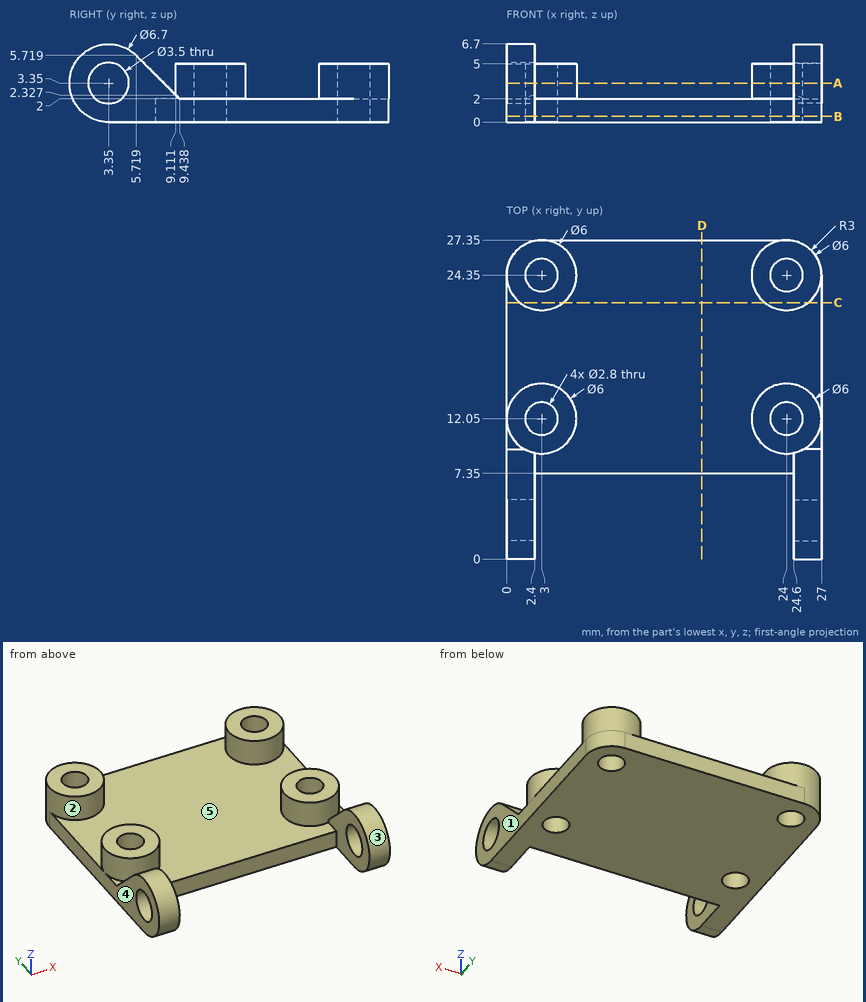
Source: three-view drawing plus pictorial views. Frame: mm from the lowest corner of the part. A direction names the side the tool comes from. Round coordinates to 2 decimals unless told otherwise and drop trailing zeros. Order: outer loops, then holes, each group sorted by start corner. A loop starts at its lowest first (then second) coordinate and runs counter-clockwise, first axis right, second up. Notation, with made-up numbers: (-22, 79) - (-6, 79) arc R17 ccw to (-6, 106) - close; hole circle Ø4 at (84.5, 76.5). An arc over 180 degrees is marked (long way). Use a Markdown table: item, result.
1. Section A-A on z = 3.35. State how many separate pieces and enclosed holes the cut face has.
Evaluation:
| item | result |
|---|---|
| separate pieces | 8 |
| enclosed holes | 4 |
2. First-contact query: pin 1 (1.7 mm diameter, centred on x = 26, y = 10.5, fed in from +Z); pin 2 (6 mm diameter, centred on x = 17.5, y = 13.5, fed in from +Z); pin 3 (1.6 mm diameter, centred on x = 17, z = 1, fed in from -Y). Flat tips, straight axial feed; report the tip coordinate or a pass-through.
Evaluation:
| item | result |
|---|---|
| pin 1 | z = 5 |
| pin 2 | z = 2 |
| pin 3 | y = 7.35 |
3. Section B-B on z = 0.5. Return the cut outline in (x, y).
Evaluation:
| item | result |
|---|---|
| outline | (0, 1.59) - (2.4, 1.59) - (2.4, 7.35) - (24.6, 7.35) - (24.6, 1.59) - (27, 1.59) - (27, 24.35) arc R3 ccw to (24, 27.35) - (3, 27.35) arc R3 ccw to (0, 24.35) - close; hole circle Ø2.8 at (3, 12.05); hole circle Ø2.8 at (3, 24.35); hole circle Ø2.8 at (24, 12.05); hole circle Ø2.8 at (24, 24.35) |
4. Mould query, pull axis Y, two halves, no side actions, for the marked faces 3, 4 and 5. Classes: +Y half, -Y half, draft (parallel to the pull), parting line (faces both ways), or undercut.
Evaluation:
| item | result |
|---|---|
| face 3 | parting line |
| face 4 | draft |
| face 5 | undercut |
5. Section C-C on y = 22. Return the cut outline in (x, z) (1 decimal).
Evaluation:
| item | result |
|---|---|
| outline | (0, 0) - (27, 0) - (27, 2) - (25.9, 2) - (25.9, 5) - (22.1, 5) - (22.1, 2) - (4.9, 2) - (4.9, 5) - (1.1, 5) - (1.1, 2) - (0, 2) - close |
6. Access query for the marked faces 1 and 2. Directions: +Z, -Z, +X, -X, +Y, -Y. A direction counts if a zero-diameter tool reaches every point of the face in a straight line with its end or side. Return the directions, or none.
Evaluation:
| item | result |
|---|---|
| face 1 | +Z, -Z, +X, +Y, -Y |
| face 2 | +Z |
7. Section D-D on x = 16.75. Return the cut outline in (y, z), then the cut area to 3 significant figures.
Evaluation:
| item | result |
|---|---|
| outline | (7.35, 0) - (27.35, 0) - (27.35, 2) - (7.35, 2) - close |
| area | 40.0 mm^2 |
8. Material intervals for probe 1 along Y at (x, z) = (24, 1.9); probe 2 along Y at (x, z) = (3, 2.15); probe 3 along Y at (x, z) = (0.7, 3.35) (1 decimal), sorted ascending.
Evaluation:
| item | result |
|---|---|
| probe 1 | 7.35 to 10.65, 13.45 to 22.95, 25.75 to 27.35 |
| probe 2 | 9.05 to 10.65, 13.45 to 15.05, 21.35 to 22.95, 25.75 to 27.35 |
| probe 3 | 0 to 1.6, 5.1 to 8.1, 10.1 to 14, 22.4 to 26.3 |
